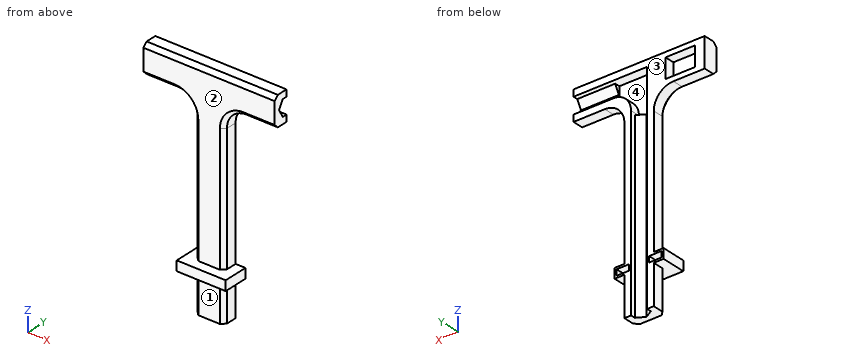
from build123d import *

# Parameters (mm, degrees)
BOSS_EXTRUDE1_DEPTH = 7.5
CUT_EXTRUDE6_DEPTH  = 5
BOSS_EXTRUDE2_START = -20
BOSS_EXTRUDE2_DEPTH = 5
CHAMFER1_SIZE       = 2
SKETCH11_W          = 15
SKETCH11_H          = 10
SKETCH11_W_2        = 6.4
SKETCH11_H_2        = 3
CUT_EXTRUDE7_DEPTH  = 5


with BuildPart() as part:
    # Sketch1 → Boss-Extrude1 (new body)
    with BuildSketch(Plane(origin=(0, 0, 0), x_dir=(1, 0, 0), z_dir=(0, 1, 0))):
        with BuildLine():
            Line((0, 0), (0, 15))
            Line((0, 15), (16, 15))
            ThreePointArc((16, 15), (23.071067812, 17.928932188), (26, 25))
            Line((26, 25), (26, 115))
            Line((26, 115), (41, 115))
            Line((41, 115), (41, 25))
            ThreePointArc((41, 25), (43.928932188, 17.928932188), (51, 15))
            Line((51, 15), (67, 15))
            Line((67, 15), (67, 0))
            Line((67, 0), (0, 0))
        make_face()
    extrude(amount=BOSS_EXTRUDE1_DEPTH)

    # Cut-Sweep1: sweep along a path in Sketch2
    with BuildLine(Plane(origin=(0, 7.5, 0), x_dir=(1, 0, 0), z_dir=(0, 1, 0))) as cut_sweep1_path:
        Line((33.5, 115), (33.5, 7.5))
        Line((33.5, 7.5), (67, 7.5))
    # Sketch3 → Cut-Sweep1 (sweep, cut)
    with BuildSketch(Plane(origin=(0, 0, -115), x_dir=(-1, 0, 0), z_dir=(0, 0, -1))):
        Polygon((-37.6, 5.132863896), (-33.5, 2.765727793), (-29.4, 5.132863896), (-29.4, 9.867136104), (-33.5, 12.234272207), (-37.6, 9.867136104), align=None)
    sweep(path=cut_sweep1_path.line, transition=Transition.RIGHT, mode=Mode.SUBTRACT)

    # Sketch7 → Cut-Extrude6 (cut)
    with BuildSketch(Plane(origin=(0, 7.5, 0), x_dir=(1, 0, 0), z_dir=(0, 1, 0))):
        with BuildLine():
            Line((47.6, 11.6), (47.6, 3.4))
            Line((47.6, 3.4), (29.4, 3.4))
            Line((29.4, 3.4), (29.4, 21.6))
            Line((29.4, 21.6), (37.6, 21.6))
            Line((37.6, 21.6), (37.6, 20.6))
            ThreePointArc((37.6, 20.6), (40.236038969, 14.236038969), (46.6, 11.6))
            Line((46.6, 11.6), (47.6, 11.6))
        make_face()
    extrude(amount=-CUT_EXTRUDE6_DEPTH, mode=Mode.SUBTRACT)

    # Sketch10 → Boss-Extrude2 (add)
    with BuildSketch(Plane(origin=(0, 0, -115), x_dir=(-1, 0, 0), z_dir=(0, 0, -1)).offset(BOSS_EXTRUDE2_START)):
        Polygon((-41, 7.5), (-46, 7.5), (-46, -5), (-21, -5), (-21, 7.5), (-26, 7.5), (-26, 0), (-41, 0), align=None)
    extrude(amount=-BOSS_EXTRUDE2_DEPTH)

    # Chamfer1
    chamfer1_edges = [part.edges().sort_by_distance(p)[0] for p in [
        (26, 0, -57.5),
        (41, 0, -105),
        (33.5, 0, 0),
        (8, 0, -15),
        (23.071067812, 0, -17.928932188),
        (26, 0, -105),
        (41, 0, -57.5),
        (43.928932188, 0, -17.928932188),
        (59, 0, -15),
    ]]
    chamfer(chamfer1_edges, length=CHAMFER1_SIZE)

    # Sketch11 → Cut-Extrude7 (cut)
    with BuildSketch(Plane(origin=(0, 7.5, 0), x_dir=(1, 0, 0), z_dir=(0, 1, 0))):
        with Locations((12.5, 7.5)):
            Rectangle(SKETCH11_W, SKETCH11_H)
        with Locations((25.2, 92.5)):
            Rectangle(SKETCH11_W_2, SKETCH11_H_2)
        with Locations((41.8, 92.5)):
            Rectangle(SKETCH11_W_2, SKETCH11_H_2)
    extrude(amount=-CUT_EXTRUDE7_DEPTH, mode=Mode.SUBTRACT)


solid = part.part
Verification items for the finished model (mm, model axes). Face numbers are marked on the shaded views. A direction names the side the tool comes from. Round coordinates to 2 decimals unless told otherwise and drop trailing zeros. Order: outer loops, then holes, each group sorted by start corner. A loop starts at its lowest first (then second) coordinate and runs counter-clockwise, first axis right, second up.
1. Thickness scan on L1, parallel to Z at x = 59.5, y = 6.75; L2, parallel to X at y = 6, z = -41; L3, parallel to X at y = 1.5, z = -94.5. Record the ranges inside material, lowest first.
Final values:
L1: z = -15 to -11.6, -3.4 to 0
L2: x = 26 to 29.4, 37.6 to 41
L3: x = 21 to 46
2. Section check A-A on x = 57. Record the cut outline in (y, z).
Final values:
outline: (0, -13) - (2, -15) - (7.5, -15) - (7.5, -11.6) - (5.13, -11.6) - (2.77, -7.5) - (5.13, -3.4) - (7.5, -3.4) - (7.5, 0) - (2, 0) - (0, -2) - close
3. Access from +Z, -Z, +X, -X, +Y, -Y to the whole of each face (thin tool, end or side, straight path). Record for the marked faces 1 and 2.
Final values:
face 1: -Z, +X, -X, -Y
face 2: +Z, +X, -X, -Y
4. Release check for a two-part mould opening along X. For the marked faces 3 and 4 record: +X half, -X half, draft (parallel to the pull), parting line (faces both ways), or undercut.
Final values:
face 3: draft
face 4: undercut
5. Section check B-B on z = -81.5. Record the cut outline in (x, y).
Final values:
outline: (26, 2) - (28, 0) - (39, 0) - (41, 2) - (41, 7.5) - (37.6, 7.5) - (37.6, 5.13) - (33.5, 2.77) - (29.4, 5.13) - (29.4, 7.5) - (26, 7.5) - close
6. Section check C-C on y = -2. Record the cut outline in (x, z).
Final values:
outline: (21, -95) - (46, -95) - (46, -90) - (21, -90) - close
7. Section check D-D on z = -9.5. Record the cut outline in (x, y).
Final values:
outline: (0, 0) - (67, 0) - (67, 3.92) - (47.6, 3.92) - (47.6, 2.5) - (29.4, 2.5) - (29.4, 7.5) - (20, 7.5) - (20, 2.5) - (5, 2.5) - (5, 7.5) - (0, 7.5) - close
8. Go/stop test with flat-tipped pins: P1, Ø2.5, axis at y = 3.5, z = -93, coming from the -X side; P2, Ø4.5, axis at x = 58, y = 3.5, coming from the -Z side; P3, Ø2, axis at y = 0, z = -78.5, coming from the +X side. Record where each tip stops, or that it passes through.
Final values:
P1: stops at x = 21
P2: stops at z = -15
P3: stops at x = 40
